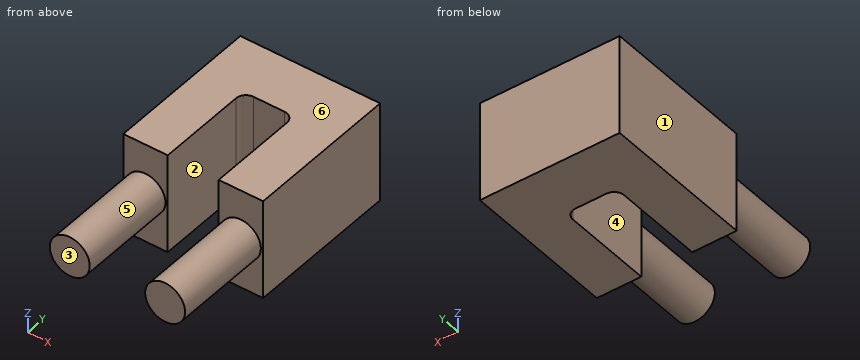
Autodesk Fusion 360 part; units mm, degrees
sketch "baza" plane through (0, 0, 0) normal (0, 0, 1) x (1, 0, 0)
  line L0 (1.275, 1.275) -> (-1.275, 1.275)
  line L1 (-1.275, 1.275) -> (-1.275, -1.275)
  line L2 (-1.275, -1.275) -> (1.275, -1.275)
  line L3 (1.275, -1.275) -> (1.275, 1.275)
  line L4 (1.275, 1.275) -> (-1.275, -1.275) construction
  line L5 (-1.275, 1.275) -> (1.275, -1.275) construction
  line L6 (3.5, 0) -> (3.5, -1.275)
  line L7 (-3.5, -1.275) -> (-3.5, 0)
  line L8 (-1.275, -1.275) -> (-3.5, -1.275)
  line L9 (1.275, -1.275) -> (3.5, -1.275)
  line L10 (3.5, 0) -> (3.5, 4)
  line L11 (3.5, 4) -> (-3.5, 4)
  line L12 (-3.5, 4) -> (-3.5, 0)
  line L13 (-1.275, -1.275) -> (-1.275, -3.725)
  line L14 (1.275, -1.275) -> (1.275, -3.725)
  line L15 (1.275, -3.725) -> (3.5, -3.725)
  line L16 (3.5, -3.725) -> (3.5, -1.275)
  line L17 (-3.5, -1.275) -> (-3.5, -3.725)
  line L18 (-3.5, -3.725) -> (-1.275, -3.725)
  line L19 (-1.275, 0.775) -> (1.275, 0.775)
  dimension "d1" = 2.55
  dimension "d4" = 7
  dimension "d11" = 7
  dimension "d12" = 4
  dimension "d16" = 1.275
  dimension "d17" = 2.45
  dimension "d18" = 0.5
extrude "Extrude1" add sketch "baza" along normal blind 5 contours L0 L1 L3 L6 L7 L8 L9 L10 L11 L12 | L9 L14 L15 L16 | L8 L13 L17 L18
sketch "dinti" plane through (0, -3.725, 0) normal (0, -1, 0) x (1, 0, 0)
  line L0 (-3.5, 0) -> (-1.275, 0)
  line L1 (-1.275, 0) -> (-1.275, 5)
  line L2 (-1.275, 5) -> (-3.5, 5)
  line L3 (-3.5, 5) -> (-3.5, 0)
  line L4 (-2.3875, 5) -> (-2.3875, 0) construction
  circle A0 centre (-2.3875, 2.5) radius 1
  line L5 (-1.275, 0) -> (1.275, 0) construction
  line L6 (1.275, 0) -> (1.275, 5) construction
  line L7 (1.275, 5) -> (-1.275, 5) construction
  line L8 (-1.275, 5) -> (-1.275, 0) construction
  line L9 (0, 5) -> (0, 0) construction
  circle A1 centre (2.3875, 2.5) radius 1
  line L10 (-3.5, 0) -> (-1.275, 0)
  line L11 (-1.275, 0) -> (-1.275, 5)
  line L12 (-1.275, 5) -> (-3.5, 5)
  line L13 (-3.5, 5) -> (-3.5, 0)
  dimension "d8" = 2
extrude "Extrude2" add sketch "dinti" along normal blind 5 contours A0 | A1
fillet "Fillet1" radius 0.5 2 edges at (1.275, 1.275, 2.5) (-1.275, 1.275, 2.5)
equation "d17 = 3.725 mm - 1.275 mm"
Check sheet for the modelled part. Datum: model origin and axes. Units: mm. Face numbers are marked on the shaded views. A direction names the side the tool comes from. Give positions to 0.01 mm unless a question says otherwise; leave off trailing zeros. Write each loop counter-clockwise with the first axis right and the second up, starting at its lowest first coordinate (ties: lowest second). Pieces come first, ordered by that corner, then holes. Notation, with made-up numbers: (20.25, 17) - (43.25, 17) arc R37 cw to (43.25, 55) - close; hole circle Ø1 at (80, 52.25). An arc over 180 degrees is marked (long way). Answer as a JSON object with one key per item and string values. Group by question number.
1) Sectioned sample at D-D (y = 1). Record the cut outline in (x, z).
2) Sectioned sample at C-C (x = -3). Record the cut outline in (y, z) (3 decimals).
3) Access from +Z, -Z, +X, -X, +Y, -Y to the whole of each face (thin tool, end or side, straight path). Record for the marked faces 4, 5 and 6.
4) Sectioned sample at A-A (y = -1.75). Record the cut outline in (x, z) (3 decimals), then the cut area to 4 significant figures.
5) Thickness scan on probe 1 along X at (y, z) = (-1.5, 1.2) (3 decimals); probe 2 along Y at (x, z) = (-3, 0.35) (3 decimals); probe 3 along X at (y, z) = (-5, 2.15). Record the ranges inside material, lowest first. Write a range as from..to.
6) Release check for a two-part mould opening along X. For the marked faces 1, 2 and 3 record: pulls with the +X half, pulls with the -X half, needs draft (parallel to the pull), parting line crosses it, or undercut.
7) Depth check by flat-ended pin: P1, Ø1.7, axis at x = 0.5, z = 2, coming from the -Y side (3 decimals). Enter the tip coordinate at first touch or a pass-through.
Geometry results:
{
 "1": {"outline": "(-3.5, 0) - (-1.22, 0) - (-1.22, 5) - (-3.5, 5) - close; (1.22, 0) - (3.5, 0) - (3.5, 5) - (1.22, 5) - close"},
 "2": {"outline": "(-8.725, 1.71) - (-3.725, 1.71) - (-3.725, 0) - (4, 0) - (4, 5) - (-3.725, 5) - (-3.725, 3.29) - (-8.725, 3.29) - close"},
 "3": {"face 4": "+Z, -Z, -Y", "face 5": "-Y", "face 6": "+Z, +X, -X, +Y, -Y"},
 "4": {"outline": "(-3.5, 0) - (-1.275, 0) - (-1.275, 5) - (-3.5, 5) - close; (1.275, 0) - (3.5, 0) - (3.5, 5) - (1.275, 5) - close", "area": "22.25 mm^2"},
 "5": {"probe 1": "x = -3.5..-1.275, 1.275..3.5", "probe 2": "y = -3.725..4", "probe 3": "x = -3.32..-1.45, 1.45..3.32"},
 "6": {"face 1": "pulls with the -X half", "face 2": "undercut", "face 3": "needs draft"},
 "7": {"P1": "stops at y = -3.725"}
}
